Source: CAD feature listing. Evaluate the final solid. Frame: model axes, mm. Give positions to 0.01 mm unless a question says otherwise; leave off trailing zeros. Order: outer loops, then holes, each group sorted by start corner. A loop starts at its lowest first (then second) coordinate and runs counter-clockwise, first axis right, second up. Notation, with made-up numbers: M -23,-5.75 L -7,-5.75 A26 ccw -7,15.25 Z; hole C 22.5,62 d10. An arc over 180 degrees is marked long. Answer as a JSON object with one key per item and string values. Group by question number.
1. Material intervals for L1, parallel to X at y = -14.5, z = 1378.5; L2, parallel to Y at x = 2, z = 1143; L3, parallel to X at y = -10, z = 147, sorted ascending. Write a range as [from, to].
2. Section query A-A (z = 1029). Output: boundary loops of the cut face in (x, y).
3. Pin query (flat end, axial travel): P1, Ø9.5, axis at x = 5, y = -14.5, coming from the +Z side; P2, Ø10, axis at x = 39, y = 1.5, coming from the +Z side; P3, Ø14, axis at x = 48, y = -2, coming from the -Z side. Return the tip coordinate at first contact, or that it passes through.
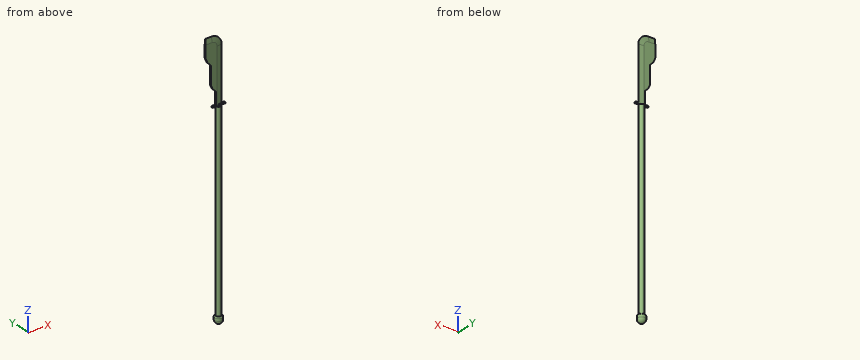
from build123d import *

# Parameters (mm, degrees)
F0_R          = 25.4
F1_DEPTH      = 1905
F2_R          = 38.1
F3_DEPTH      = 76.2
F4_W          = 50.8
F4_H          = 254
F5_DEPTH      = 6.35
F5_DEPTH_BACK = 6.35
F6_SIZE       = 50.79999
F7_R          = 101.6
F8_SIZE2      = 51.71659
F8_SIZE       = 6.34999
F9_SIZE       = 25.4
F11_R         = 38.1


# Not quite as in the source:
# - a fillet or chamfer that OpenCascade refuses, or shapes differently, is made with other operations: its cross-section is extruded or revolved along the edge and cut away or added
# - a fillet or chamfer is up to 0.001 mm smaller than in the source, because OpenCascade refuses the exact size


with BuildPart() as f1:
    # F0 (on Top) → F1 (new body)
    with BuildSketch(Plane.XY):
        Circle(F0_R)
    extrude(amount=F1_DEPTH)

    # F2 (on face) → F3 (join)
    with BuildSketch(Plane(origin=(0, 0, 0), x_dir=(1, 0, 0), z_dir=(0, 0, -1))):
        Circle(F2_R)
    extrude(amount=F3_DEPTH)

    # F4 (on Front) → F5 (join, two sides)
    with BuildSketch(Plane.XZ) as f5_sk:
        Polygon((-25.4, 1905), (0, 1905), (25.4, 1905), (63.5, 1905), (63.5, 1917.7), (31.75, 1917.7), (0, 1917.7), (-31.75, 1917.7), (-63.5, 1917.7), (-63.5, 1905), align=None)
        Polygon((0, 1917.7), (31.75, 1917.7), (31.75, 2552.7), (-31.75, 2552.7), (-31.75, 2298.7), (-31.75, 2044.7), (-31.75, 1917.7), align=None)
        with Locations((-57.15, 2171.7)):
            Rectangle(F4_W, F4_H)
        Polygon((-31.75, 2298.7), (-31.75, 2552.7), (-133.35, 2552.7), (-133.35, 2298.7), (-82.55, 2298.7), align=None)
    extrude(amount=F5_DEPTH)
    extrude(f5_sk.sketch, amount=-F5_DEPTH_BACK)

    # F6 (size 50.8 in the source; OpenCascade refuses exactly that, so slightly less here)
    f6_edges = [f1.edges().sort_by_distance(p)[0] for p in [
        (-133.35, 0, 2298.7),
        (-82.55, 0, 2044.7),
    ]]
    chamfer(f6_edges, length=F6_SIZE)

    # F7
    f7_edges = [f1.edges().sort_by_distance(p)[0] for p in [
        (31.75, 0, 2552.7),
    ]]
    fillet(f7_edges, radius=F7_R)

    # F8 (size 6.35 and 51.7165998176 in the source; OpenCascade refuses exactly that, so slightly less here)
    f8_edges = [f1.edges().sort_by_distance(p)[0] for p in [
        (31.75, 6.35, 2184.4),
        (31.75, -6.35, 2184.4),
    ]]
    f8_side = f1.faces().sort_by_distance((31.75, 0, 2184.4))[0]
    chamfer(f8_edges, length=F8_SIZE, length2=F8_SIZE2, reference=f8_side)

    # F9
    f9_edges = [f1.edges().sort_by_distance(p)[0] for p in [
        (-133.35, 0, 2349.49999),
        (-82.55, 0, 2095.49999),
    ]]
    chamfer(f9_edges, length=F9_SIZE)

    # F10: fillet of radius 12.7 on 1 edges, made by hand

    # F10_s1 → F10_t2 (revolve, cut)
    with BuildSketch(Plane.XZ):
        with BuildLine():
            ThreePointArc((25.4, 0), (34.3802561211, -3.7197438789), (38.1, -12.7))
            Line((38.1, -12.7), (38.1, 0))
            Line((38.1, 0), (25.4, 0))
        make_face()
    revolve(axis=Axis((0, 0, 0), (0, 0, -1)), mode=Mode.SUBTRACT)

    # F11
    f11_edges = [f1.edges().sort_by_distance(p)[0] for p in [
        (-38.1, 0, -76.2),
    ]]
    fillet(f11_edges, radius=F11_R)


solid = f1.part
Answer sheet:
{
 "1": {"L1": "[-20.85, 20.85]", "L2": "[-25.32, 25.32]", "L3": "[-23.35, 23.35]"},
 "2": {"outline": "C 0,0 d50.8"},
 "3": {"P1": "z = 1905", "P2": "z = 1917.7", "P3": "z = 1905"}
}
